CAD build for the part. Positions are in the model's coordinates, mm. Face numbers are marked on the shaded views. A direction names the side the tool comes from. Give positions to 0.01 mm unless a question says otherwise; leave off trailing zeros. Write each loop counter-clockwise with the first axis right and the second up, starting at its lowest first coordinate (ties: lowest second). Pieces come first, ordered by that corner, then holes. Notation, with made-up numbers: (18, -31.75) - (43, -31.75) arc R35 ccw to (43, 5.25) - close; hole circle Ø10 at (9.5, 44). An arc over 180 degrees is marked (long way). Put each result on its own line as item: value. Start each with the question number.
1. Drop flat-ended pins along their axis: pin 1 (4 mm diameter, centred on x = 32.14, y = 38.3, fed in from +Z); pin 2 (1.5 mm diameter, centred on y = -4, z = 9.5, fed in from -X); pin 3 (3 mm diameter, centred on x = 21.5, z = 5.5, fed in from +Y); pin 4 (2.5 mm diameter, centred on x = -8.68, y = -49.24, fed in from -Z). Give the stop position or say it passes through.
2. Cut at A-A on z = 10. List the corners of the cut face in (x, y), and give its area (3 significant figures).
3. Wall check: line 1 (Y direction, x = 32, z = 2.5); line 2 (Y direction, x = 0, z = 1.5); line 3 (Y direction, x = -50, z = 1). Give the ranges that are in metal, low to high.
4. Cut at B-B on y = -25. List the corners of the cut face in (x, z).
5. Cut at C-C on x = -13. List the corners of the cut face in (y, z).
6. Tool access for the marked faces 1, 2 and 3: list every direction of +Z, -Z, +X, -X, +Y, -Y with a clear straight run to the whole face (end or side of a thin tool).
from build123d import *

# Parameters (mm, degrees)
F0_R     = 60
F0_R_2   = 1.5
F1_DEPTH = 3
F2_R     = 26.5
F3_DEPTH = 25
F4_R     = 30
F4_R_2   = 26.5
F5_DEPTH = 10
F7_DEPTH = 10


with BuildPart() as f1:
    # F0 (on Top) → F1 (new body)
    with BuildSketch(Plane.XY):
        Circle(F0_R)
        with Locations((-32.1393804843, -38.3022221559)):
            Circle(F0_R_2, mode=Mode.SUBTRACT)
        with Locations((-38.3022221559, -32.1393804843)):
            Circle(F0_R_2, mode=Mode.SUBTRACT)
        with Locations((-17.1010071663, -46.9846310393)):
            Circle(F0_R_2, mode=Mode.SUBTRACT)
        with Locations((-8.6824088833, -49.2403876506)):
            Circle(F0_R_2, mode=Mode.SUBTRACT)
        with Locations((-25, -43.3012701892)):
            Circle(F0_R_2, mode=Mode.SUBTRACT)
        with Locations((-46.9846310393, -17.1010071663)):
            Circle(F0_R_2, mode=Mode.SUBTRACT)
        with Locations((-43.3012701892, -25)):
            Circle(F0_R_2, mode=Mode.SUBTRACT)
        with Locations((-49.2403876506, -8.6824088833)):
            Circle(F0_R_2, mode=Mode.SUBTRACT)
        with Locations((0, -50)):
            Circle(F0_R_2, mode=Mode.SUBTRACT)
        with Locations((8.6824088833, -49.2403876506)):
            Circle(F0_R_2, mode=Mode.SUBTRACT)
        with Locations((17.1010071663, -46.9846310393)):
            Circle(F0_R_2, mode=Mode.SUBTRACT)
        with Locations((25, -43.3012701892)):
            Circle(F0_R_2, mode=Mode.SUBTRACT)
        with Locations((32.1393804843, -38.3022221559)):
            Circle(F0_R_2, mode=Mode.SUBTRACT)
        with Locations((38.3022221559, -32.1393804843)):
            Circle(F0_R_2, mode=Mode.SUBTRACT)
        with Locations((43.3012701892, -25)):
            Circle(F0_R_2, mode=Mode.SUBTRACT)
        with Locations((46.9846310393, -17.1010071663)):
            Circle(F0_R_2, mode=Mode.SUBTRACT)
        with Locations((49.2403876506, -8.6824088833)):
            Circle(F0_R_2, mode=Mode.SUBTRACT)
        with Locations((-50, 0)):
            Circle(F0_R_2, mode=Mode.SUBTRACT)
        with Locations((-49.2403876506, 8.6824088833)):
            Circle(F0_R_2, mode=Mode.SUBTRACT)
        with Locations((-46.9846310393, 17.1010071663)):
            Circle(F0_R_2, mode=Mode.SUBTRACT)
        with Locations((-43.3012701892, 25)):
            Circle(F0_R_2, mode=Mode.SUBTRACT)
        with Locations((-38.3022221559, 32.1393804843)):
            Circle(F0_R_2, mode=Mode.SUBTRACT)
        with Locations((-32.1393804843, 38.3022221559)):
            Circle(F0_R_2, mode=Mode.SUBTRACT)
        with Locations((-25, 43.3012701892)):
            Circle(F0_R_2, mode=Mode.SUBTRACT)
        with Locations((-17.1010071663, 46.9846310393)):
            Circle(F0_R_2, mode=Mode.SUBTRACT)
        with Locations((-8.6824088833, 49.2403876506)):
            Circle(F0_R_2, mode=Mode.SUBTRACT)
        with Locations((50, 0)):
            Circle(F0_R_2, mode=Mode.SUBTRACT)
        with Locations((49.2403876506, 8.6824088833)):
            Circle(F0_R_2, mode=Mode.SUBTRACT)
        with Locations((43.3012701892, 25)):
            Circle(F0_R_2, mode=Mode.SUBTRACT)
        with Locations((46.9846310393, 17.1010071663)):
            Circle(F0_R_2, mode=Mode.SUBTRACT)
        with Locations((25, 43.3012701892)):
            Circle(F0_R_2, mode=Mode.SUBTRACT)
        with Locations((0, 50)):
            Circle(F0_R_2, mode=Mode.SUBTRACT)
        with Locations((8.6824088833, 49.2403876506)):
            Circle(F0_R_2, mode=Mode.SUBTRACT)
        with Locations((17.1010071663, 46.9846310393)):
            Circle(F0_R_2, mode=Mode.SUBTRACT)
        with Locations((38.3022221559, 32.1393804843)):
            Circle(F0_R_2, mode=Mode.SUBTRACT)
        with Locations((32.1393804843, 38.3022221559)):
            Circle(F0_R_2, mode=Mode.SUBTRACT)
    extrude(amount=F1_DEPTH)

    # F2 (on face) → F3 (cut)
    with BuildSketch(Plane.XY.offset(3)):
        Circle(F2_R)
    extrude(amount=-F3_DEPTH, mode=Mode.SUBTRACT)

    # F4 (on face) → F5 (join)
    with BuildSketch(Plane.XY.offset(3)):
        Circle(F4_R)
        Circle(F4_R_2, mode=Mode.SUBTRACT)
    extrude(amount=F5_DEPTH)

    # F6 (on face) → F7 (join)
    with BuildSketch(Plane.XY.offset(3)):
        with BuildLine():
            ThreePointArc((-19.843134833, -22.5), (-21.2132034356, -21.2132034356), (-22.5, -19.843134833))
            Line((-22.5, -19.843134833), (-22.5, -22.5))
            Line((-22.5, -22.5), (-19.843134833, -22.5))
        make_face()
        with BuildLine():
            Line((22.5, -22.5), (22.5, -19.843134833))
            ThreePointArc((22.5, -19.843134833), (21.2132034356, -21.2132034356), (19.843134833, -22.5))
            Line((19.843134833, -22.5), (22.5, -22.5))
        make_face()
        with BuildLine():
            Line((22.5, 19.843134833), (22.5, 22.5))
            Line((22.5, 22.5), (19.843134833, 22.5))
            ThreePointArc((19.843134833, 22.5), (21.2132034356, 21.2132034356), (22.5, 19.843134833))
        make_face()
        with BuildLine():
            ThreePointArc((-22.5, 19.843134833), (-21.2132034356, 21.2132034356), (-19.843134833, 22.5))
            Line((-19.843134833, 22.5), (-22.5, 22.5))
            Line((-22.5, 22.5), (-22.5, 19.843134833))
        make_face()
    extrude(amount=F7_DEPTH)


solid = f1.part
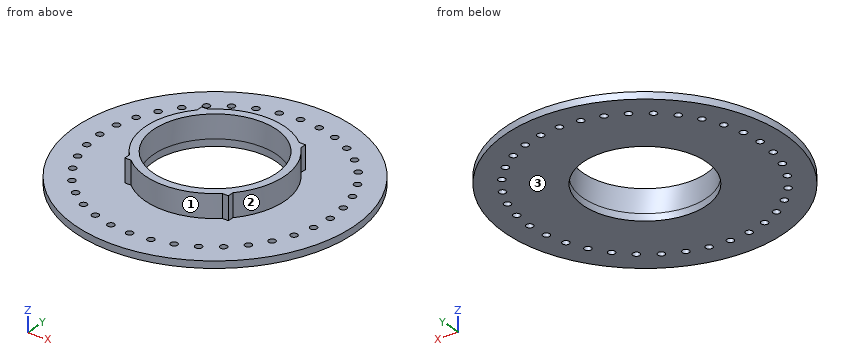
Report:
1. pin 1: stops at z = 3
1. pin 2: stops at x = -29.82
1. pin 3: stops at y = 22.5
1. pin 4: passes through
2. outline: (-22.5, -22.5) - (-19.84, -22.5) arc R30 ccw to (19.84, -22.5) - (22.5, -22.5) - (22.5, -19.84) arc R30 ccw to (22.5, 19.84) - (22.5, 22.5) - (19.84, 22.5) arc R30 ccw to (-19.84, 22.5) - (-22.5, 22.5) - (-22.5, 19.84) arc R30 ccw to (-22.5, -19.84) - close; hole circle Ø53 at (0, 0)
2. area: 635 mm²
3. line 1: y = -50.75 to -39.8, -36.81 to 36.81, 39.8 to 50.75
3. line 2: y = -60 to -51.5, -48.5 to -26.5, 26.5 to 48.5, 51.5 to 60
3. line 3: y = -33.17 to -9.98, -7.39 to -1.5, 1.5 to 7.39, 9.98 to 33.17
4. outline: (-54.54, 0) - (-44.8, 0) - (-44.8, 3) - (-54.54, 3) - close; (-41.8, 0) - (-8.79, 0) - (-8.79, 13) - (-16.58, 13) - (-16.58, 3) - (-41.8, 3) - close; (8.79, 0) - (41.8, 0) - (41.8, 3) - (16.58, 3) - (16.58, 13) - (8.79, 13) - close; (44.8, 0) - (54.54, 0) - (54.54, 3) - (44.8, 3) - close
5. outline: (-58.57, 0) - (-23.09, 0) - (-23.09, 13) - (-27.04, 13) - (-27.04, 3) - (-58.57, 3) - close; (23.09, 0) - (58.57, 0) - (58.57, 3) - (27.04, 3) - (27.04, 13) - (23.09, 13) - close
6. face 1: +Z, -Y
6. face 2: +Z, +X
6. face 3: -Z, +X, -X, +Y, -Y
